Autodesk Fusion 360 part; units mm, degrees
sketch "PinWay" plane through (0, 65, 0) normal (0, 1, 0) x (1, 0, 0)
  line L0 (0, 0) -> (0, -30) construction
  line L1 (0, -30) -> (4.125, -30)
  line L2 (4.125, -30) -> (4.125, -25.8571)
  line L3 (-4.125, -30) -> (-4.125, -25.8571)
  line L4 (0, -30) -> (-4.125, -30)
  arc A0 (4.125, -25.8571) -> (-4.125, -25.8571) centre (0, -21.5) ccw
  circle A1 centre (0, -21.5) radius 5.5
  circle A2 centre (0, -21.5) radius 3
  dimension "d1" = 0
  dimension "d2" = 0
  dimension "d3" = 0
  dimension "d4" = 0
  dimension "d5" = 11
  dimension "d6" = 0
extrude "Extrude1" add sketch "PinWay" against normal blind 49 contours A2
extrude "Extrude2" cut sketch "PinWay" against normal blind 24 contours A2
sketch "Sketch6" plane through (0, 16, 0) normal (0, -1, 0) x (1, 0, 0)
  circle A0 centre (0, 21.5) radius 3
  circle A1 centre (0, 21.5) radius 5.5
  dimension "d171" = 11
sketch "Sketch7" plane through (0, 41, 0) normal (0, 1, 0) x (-1, 0, 0)
  circle A0 centre (0, 21.5) radius 3
  circle A1 centre (0, 21.5) radius 5.5
extrude "Extrude3" add sketch "Sketch6" against normal blind 6
extrude "Extrude4" add sketch "Sketch7" against normal blind 6
chamfer "Chamfer3" distance 0.8 angle 45 2 edges at (-5.1278, 16, 19.5111) (5.1278, 41, 19.5111)
chamfer "Chamfer4" distance 0.4 angle 45 2 edges at (-5.1278, 22, 23.4889) (5.1278, 35, 23.4889)
chamfer "Chamfer1" [suppressed]
chamfer "Chamfer2" [suppressed]
equation "d167 = TopPinBlank"
equation "d169 = TopPinBlank + TopPinLength"
equation "d171 = Pin"
equation "d173 = -1 * SpoolPinEnds"
equation "d175 = -1 * SpoolPinEnds"
equation "Pin = 11 mm"
equation "TopPinLength = 25 mm"
equation "TopPinBlank = -49 mm"
equation "SpoolPinEnds = 6 mm"
equation "d1 = PinWayDiameter"
equation "d2 = PinWayDepth"
equation "d3 = BodyThickness"
equation "d4 = PinWayOpening / 2"
equation "d5 = Pin"
equation "d6 = SpoolPinCenter"
Source: CAD feature listing. Evaluate the final solid. Frame: model axes, mm. A direction names the side the tool comes from. Round coordinates to 2 decimals unless told otherwise and drop trailing zeros. Loops run counter-clockwise (first coordinate to the right, second up) from the corner with the lowest first, then second, coordinate; pieces in that order, holes last. Notation, with made-up numbers: M -23,-32.75 L 35,-32.75 A30 cw 35,0.25 Z; hole C -32,33 d4. An arc over 180 degrees is marked long. Use a Markdown table: item, result. Add a question column.
1. Line query: line 1 (Y direction, x = -2, z = 25.5); line 2 (Y direction, x = 2, z = 26.5); line 3 (X direction, y = 24.5, z = 21.25). Output: solid intervals per line, ascending.
2. Mould query, pull axis Y, two halves, no side actions, for faces 1 (the cylindrical face through (-0.65, 28.59, 24.43)), 2 (the cylindrical face through (0.716, 37.834, 26.953)), 3 (the flat face through (0, 41, 22)). Classes: pulls with the +Y half, pulls with the -Y half, needs draft (parallel to the pull), parting line crosses it, or undercut.
3. Contact query for flat-ended pins moving along their axis: P1, Ø1.5, axis at y = 29.5, z = 20, coming from the +X side; P2, Ø1, axis at x = -2, y = 20.5, coming from the -Z side; P3, Ø5, axis at x = 2, y = 30.5, coming from the +Z side. Output: stop coordinate, or through.
4. Section query A-A on x = 0. Return the cut outline in (y, z).
5. Reachability of faces 4 (the flat face through (2, 22, 19)), 5 (the cylindrical face through (-0.716, 19.166, 26.953)) from +Z, -Z, +X, -X, +Y, -Y: full face, straight path, thin tool, end or side. Return the list, or none.
6. Section query B-B on y = 24.5. Return the cut outline in (x, z).
Reported:
| question | item | result |
|---|---|---|
| 1 | line 1 | y = 16 to 22, 35 to 41 |
| 1 | line 2 | y = 16.69 to 21.71, 35.29 to 40.31 |
| 1 | line 3 | x = -2.99 to 2.99 |
| 2 | face 1 | undercut |
| 2 | face 2 | needs draft |
| 2 | face 3 | pulls with the +Y half |
| 3 | P1 | stops at x = 2.9 |
| 3 | P2 | stops at z = 16.21 |
| 3 | P3 | stops at z = 24.5 |
| 4 | outline | M 16,16.8 L 16.8,16 L 21.6,16 L 22,16.4 L 22,18.5 L 35,18.5 L 35,16.4 L 35.4,16 L 40.2,16 L 41,16.8 L 41,26.2 L 40.2,27 L 35.4,27 L 35,26.6 L 35,24.5 L 22,24.5 L 22,26.6 L 21.6,27 L 16.8,27 L 16,26.2 Z |
| 5 | face 4 | none |
| 5 | face 5 | +Y, -Y |
| 6 | outline | C 0,21.5 d6 |
